Autodesk Inventor part; units mm, degrees
ref_plane "YZ Plane" through (0, 0, 0) normal (1, 0, 0) x (0, 1, 0)
ref_plane "XZ Plane" through (0, 0, 0) normal (0, 1, 0) x (-1, 0, 0)
ref_plane "XY Plane" through (0, 0, 0) normal (0, 0, 1) x (1, 0, 0)
sketch "Sketch1" plane through (0, 0, 0) normal (0, 1, 0) x (-1, 0, 0)
  arc A0 (-85.6318, 54.0093) -> (-85.4518, 52.6798) centre (-90.4518, 52.6798) ccw
  line L0 (-85.6318, 54.0093) -> (-85.6318, 82.6798)
  line L1 (-85.6318, 82.6798) -> (-75.8236, 82.6798)
  line L2 (-75.8236, 82.6798) -> (-75.8236, 52.6798)
  line L3 (-75.8236, 52.6798) -> (-85.4518, 52.6798)
  circle A1 centre (89.5482, 282.6798) radius 5
  circle A2 centre (-90.4518, 282.6798) radius 5
  circle A3 centre (89.5482, 52.6798) radius 5
  circle A4 centre (-15.4518, 247.6798) radius 5
  circle A5 centre (94.5482, 87.6798) radius 5
  circle A6 centre (-15.4518, 87.6798) radius 5
  circle A7 centre (14.5482, 247.6798) radius 5
  circle A8 centre (-95.4518, 247.6798) radius 5
  circle A9 centre (14.5482, 87.6798) radius 5
  circle A10 centre (-95.4518, 87.6798) radius 5
  circle A11 centre (94.5482, 247.6798) radius 5
  line L4 (-25.6318, 52.6798) -> (-35.3318, 52.6798)
  line L5 (-35.3318, 52.6798) -> (-35.3318, 82.6798)
  line L6 (-35.3318, 82.6798) -> (-25.6318, 82.6798)
  line L7 (-25.6318, 82.6798) -> (-25.6318, 52.6798)
  line L8 (24.3682, 82.6798) -> (34.1764, 82.6798)
  line L9 (34.1764, 82.6798) -> (34.1764, 52.6798)
  line L10 (34.1764, 52.6798) -> (24.3682, 52.6798)
  line L11 (24.3682, 52.6798) -> (24.3682, 82.6798)
  line L12 (84.3682, 52.6798) -> (74.6682, 52.6798)
  line L13 (74.6682, 52.6798) -> (74.6682, 82.6798)
  line L14 (74.6682, 82.6798) -> (84.3682, 82.6798)
  line L15 (84.3682, 82.6798) -> (84.3682, 52.6798)
  arc A12 (86.1572, 45.1798) -> (96.0053, 53.4434) centre (86.1572, 55.1798) ccw
  line L16 (96.0053, 53.4434) -> (115.8421, 165.9434)
  arc A13 (115.8421, 165.9434) -> (115.8421, 169.4163) centre (105.994, 167.6798) ccw
  line L17 (115.8421, 169.4163) -> (96.0053, 281.9163)
  arc A14 (96.0053, 281.9163) -> (86.1572, 290.1798) centre (86.1572, 280.1798) ccw
  line L18 (86.1572, 290.1798) -> (-87.0608, 290.1798)
  arc A15 (-87.0608, 290.1798) -> (-96.9089, 281.9163) centre (-87.0608, 280.1798) ccw
  line L19 (-96.9089, 281.9163) -> (-116.7457, 169.4163)
  arc A16 (-116.7457, 169.4163) -> (-116.7457, 165.9434) centre (-106.8976, 167.6798) ccw
  line L20 (-116.7457, 165.9434) -> (-96.9089, 53.4434)
  arc A17 (-96.9089, 53.4434) -> (-87.0608, 45.1798) centre (-87.0608, 55.1798) ccw
  line L21 (-87.0608, 45.1798) -> (86.1572, 45.1798)
  line L22 (12.0482, 180.1798) -> (12.0482, 155.1798)
  line L23 (12.0482, 155.1798) -> (-12.9518, 155.1798)
  line L24 (-12.9518, 155.1798) -> (-12.9518, 180.1798)
  line L25 (-12.9518, 180.1798) -> (12.0482, 180.1798)
  circle A18 centre (25.0482, 100.1798) radius 1.5
  circle A19 centre (25.0482, 230.1798) radius 1.5
  circle A20 centre (-86.9518, 230.1798) radius 1.5
  circle A21 centre (-25.9518, 149.1798) radius 1.5
  circle A22 centre (-25.9518, 100.1798) radius 1.5
  line L26 (-22.4518, 167.6798) -> (-22.4518, 162.6798)
  line L27 (-22.4518, 162.6798) -> (-90.4518, 162.6798)
  line L28 (-90.4518, 162.6798) -> (-90.4518, 167.6798)
  line L29 (-90.4518, 167.6798) -> (-22.4518, 167.6798)
  circle A23 centre (-25.9518, 230.1798) radius 1.5
  circle A24 centre (25.0482, 181.1798) radius 1.5
  circle A25 centre (25.0482, 149.1798) radius 1.5
  circle A26 centre (86.0482, 100.1798) radius 1.5
  circle A27 centre (86.0482, 230.1798) radius 1.5
  circle A28 centre (-86.9518, 181.1798) radius 1.5
  circle A29 centre (-86.9518, 149.1798) radius 1.5
  circle A30 centre (-86.9518, 100.1798) radius 1.5
  circle A31 centre (-25.9518, 181.1798) radius 1.5
  line L30 (89.5482, 167.6798) -> (89.5482, 162.6798)
  line L31 (89.5482, 162.6798) -> (21.5482, 162.6798)
  line L32 (21.5482, 162.6798) -> (21.5482, 167.6798)
  line L33 (21.5482, 167.6798) -> (89.5482, 167.6798)
  circle A32 centre (86.0482, 181.1798) radius 1.5
  circle A33 centre (86.0482, 149.1798) radius 1.5
  circle A34 centre (-65.4518, 267.6798) radius 4
  circle A35 centre (-65.4518, 67.6798) radius 4
  circle A36 centre (64.5482, 267.6798) radius 4
  circle A37 centre (64.5482, 67.6798) radius 4
  point P0 (0, 0)
extrude "Extrusion1" add sketch "Sketch1" along normal blind 5 contours L0 L1 L2 L3 A0 | A1 | A2 | A3 | A4 | A5 | A6 | A7 | A8 | A9 | A10 | A11 | L4 L5 L6 L7 | L8 L9 L10 L11 | L12 L13 L14 L15 | L21 A17 L20 A16 L19 A15 L18 A14 L17 A13 L16 A12 | L22 L23 L24 L25 | A18 | A19 | A20 | A21 | A22 | L26 L27 L28 L29 | A23 | A24 | A25 | A26 | A27 | A28 | A29 | A30 | A31 | L30 L31 L32 L33 | A32 | A33 | A34 | A35 | A36 | A37
sketch "Sketch2" plane through (0, 5, 0) normal (0, 1, 0) x (1, 0, 0)
  arc A0 (85.6318, -54.0093) -> (85.4518, -52.6798) centre (90.4518, -52.6798) ccw
  circle A1 centre (90.4518, -282.6798) radius 5
  circle A2 centre (-89.5482, -52.6798) radius 5
  circle A3 centre (-89.5482, -282.6798) radius 5
  circle A4 centre (90.4518, -52.6798) radius 5
  point P0 (0, 0)
extrude "Extrusion2" cut sketch "Sketch2" against normal through all
sketch "Sketch3" plane through (0, 5, 0) normal (0, 1, 0) x (1, 0, 0)
  line L0 (12.9518, -180.1798) -> (12.9518, -155.1798)
  line L1 (12.9518, -155.1798) -> (-12.0482, -155.1798)
  line L2 (-12.0482, -155.1798) -> (-12.0482, -180.1798)
  line L3 (-12.0482, -180.1798) -> (12.9518, -180.1798)
  point P0 (0, 0)
extrude "Extrusion3" cut sketch "Sketch3" against normal mid plane 50
sketch "Sketch4" plane through (0, 5, 0) normal (0, 1, 0) x (1, 0, 0)
  line L0 (-12.0482, -155.1798) -> (-12.0482, -180.1798)
  line L1 (-12.0482, -180.1798) -> (82.9518, -180.1798)
  line L2 (82.9518, -180.1798) -> (82.9518, -60.1798)
  line L3 (82.9518, -60.1798) -> (-12.0482, -60.1798)
  line L4 (-12.0482, -60.1798) -> (-12.0482, -180.1798)
  line L5 (12.9518, -180.1798) -> (12.9518, -155.1798)
  line L6 (12.9518, -180.1798) -> (-82.0482, -180.1798)
  line L7 (-82.0482, -180.1798) -> (-82.0482, -60.1798)
  line L8 (-82.0482, -60.1798) -> (12.9518, -60.1798)
  line L9 (12.9518, -60.1798) -> (12.9518, -180.1798)
  line L10 (82.9518, -60.1798) -> (-82.0482, -60.1798)
  line L11 (-82.0482, -60.1798) -> (-82.0482, -57.6798)
  line L12 (-82.0482, -57.6798) -> (82.9518, -57.6798)
  line L13 (82.9518, -57.6798) -> (82.9518, -60.1798)
  line L14 (-82.0482, -57.6798) -> (-79.5482, -57.6798)
  line L15 (-79.5482, -57.6798) -> (-79.5482, -180.1798)
  line L16 (-79.5482, -180.1798) -> (-82.0482, -180.1798)
  line L17 (-82.0482, -180.1798) -> (-82.0482, -57.6798)
  line L18 (82.9518, -180.1798) -> (80.4518, -180.1798)
  line L19 (80.4518, -180.1798) -> (80.4518, -57.6798)
  line L20 (80.4518, -57.6798) -> (82.9518, -57.6798)
  line L21 (82.9518, -57.6798) -> (82.9518, -180.1798)
  line L22 (82.9518, -180.1798) -> (-82.0482, -180.1798)
  line L23 (-82.0482, -180.1798) -> (-82.0482, -182.6798)
  line L24 (-82.0482, -182.6798) -> (82.9518, -182.6798)
  line L25 (82.9518, -182.6798) -> (82.9518, -180.1798)
  point P0 (0, 0)
  point P1 (-79.5482, -60.1798)
  point P2 (-12.0482, -60.1798)
  point P3 (80.4518, -60.1798)
  dimension "d6" = 95
  dimension "d7" = 120
  dimension "d8" = 95
  dimension "d9" = 120
  dimension "d10" = 2.5
  dimension "d11" = 2.5
  dimension "d12" = 2.5
  dimension "d13" = 2.5
extrude "Extrusion4" add sketch "Sketch4" along normal blind 50 contours L1 L25 L24 L23 L6 | L8 L15 L12 L19 L3 | L6 L7 L8 L15 | L8 L11 L12 L15 | L19 L3 L2 L1 | L19 L12 L13 L3
sketch "Sketch6" plane through (80.4518, 5, 60.1798) normal (-1, 0, 0) x (0, 0, 1)
  line L0 (122.5, 0) -> (0, 0)
  line L1 (122.5, 0) -> (122.5, 50)
  line L2 (0, 50) -> (122.5, 50)
  line L3 (0, 0) -> (0, 50)
  line L4 (120, 0) -> (120, 50)
  line L5 (0, 0) -> (0, 50)
  line L6 (0, 0) -> (120, 0)
  line L7 (120, 0) -> (120, 5)
  line L8 (120, 5) -> (0, 5)
  line L9 (0, 5) -> (0, 0)
  line L10 (0, 5) -> (120, 0)
  point P0 (-60.1798, -5)
  dimension "d26" = 5
extrude "Extrusion6" add sketch "Sketch6" along normal up to surface (160 mm away) contours L0 L3 L10
sketch "Sketch7" plane through (-79.5482, 10, 60.1798) normal (0, 0.9991, 0.0416) x (1, 0, 0)
  line L0 (67.5, -120.1041) -> (67.5, -95.1258)
  line L1 (67.5, -95.1258) -> (92.5, -95.1258)
  line L2 (92.5, -95.1258) -> (92.5, -120.1041)
  line L3 (160, -118.0226) -> (0, -118.0226)
  point P0 (79.5482, 59.7114)
  point P1 (67.5, -118.0226)
  point P2 (92.5, -118.0226)
extrude "Extrusion7" cut sketch "Sketch7" against normal blind 10
sketch "Sketch8" plane through (-86.1572, 0, 290.1798) normal (0, 0, 1) x (1, 0, 0)
  line L0 (0, 0) -> (173.218, 0)
  line L1 (173.218, 0) -> (173.218, 5)
  line L2 (0, 5) -> (173.218, 5)
  line L3 (0, 0) -> (0, 5)
  line L4 (173.218, 0) -> (173.218, 5)
  line L5 (173.218, 0) -> (115.5513, 0)
  line L6 (115.5513, 0) -> (57.8843, 0)
  line L7 (0, 0) -> (173.218, 0)
  line L8 (0, 0) -> (-9.8481, 0)
  line L9 (0, 0) -> (57.667, 0)
  line L10 (57.667, 0) -> (57.667, 5)
  line L11 (0, 5) -> (173.218, 5)
  line L12 (115.5513, 0) -> (115.5513, 5)
  line L13 (99.109, 5) -> (166.609, 5)
  line L14 (55.167, 7.5) -> (60.167, 7.5)
  line L15 (60.167, 7.5) -> (60.167, 2.5)
  line L16 (60.167, 2.5) -> (55.167, 2.5)
  line L17 (55.167, 2.5) -> (55.167, 7.5)
  line L18 (55.167, 7.5) -> (60.167, 2.5) construction
  line L19 (60.167, 7.5) -> (55.167, 2.5) construction
  line L20 (113.0513, 7.5) -> (118.0513, 7.5)
  line L21 (118.0513, 7.5) -> (118.0513, 2.5)
  line L22 (118.0513, 2.5) -> (113.0513, 2.5)
  line L23 (113.0513, 2.5) -> (113.0513, 7.5)
  line L24 (113.0513, 7.5) -> (118.0513, 2.5) construction
  line L25 (118.0513, 7.5) -> (113.0513, 2.5) construction
  line L26 (60.167, 2.5) -> (62.667, 2.5)
  line L27 (62.667, 2.5) -> (60.167, 5)
  line L28 (55.167, 2.5) -> (52.667, 2.5)
  line L29 (52.667, 2.5) -> (55.167, 5)
  line L30 (118.0513, 2.5) -> (120.5513, 2.5)
  line L31 (120.5513, 2.5) -> (118.0513, 5)
  line L32 (113.0513, 2.5) -> (110.5513, 2.5)
  line L33 (110.5513, 2.5) -> (113.0513, 5)
  point P0 (86.1572, 0)
  dimension "d31" = 57.6667
  dimension "d33" = 57.667
  dimension "d34" = 5
  dimension "d35" = 5
  dimension "d36" = 5
  dimension "d37" = 5
  dimension "d38" = 2.5
  dimension "d39" = 2.5
  dimension "d40" = 2.5
  dimension "d41" = 2.5
extrude "Extrusion8" cut sketch "Sketch8" against normal up to surface (107.5 mm away) contours L16 L17 L2 L10 | L10 L2 L15 L16 | L17 L28 L29 | L15 L27 L26 | L22 L23 L2 L12 | L12 L2 L21 L22 | L21 L31 L30 | L32 L33 L23
properties part number "upper base"
Part model, mm, in its own coordinate system. A direction names the side the tool comes from. Coordinates: 2 decimals unless noted, no trailing zeros. Loops run counter-clockwise (first coordinate to the right, second up) from the corner with the lowest first, then second, coordinate; pieces in that order, holes last. Notation, with made-up numbers: M 54,5 L 94,5 A23 ccw 94,22 Z; hole C 29.5,-20.75 d11. An arc over 180 degrees is marked long. Use a Markdown table: item, result. Add a question column.
Q1. Cut at A-A (y = 33). Write the cut outline in (x, z), and give its area (4 significant figures).
Q2. Which spindle directions (+Z, -Z, +X, -X, +Y, -Y) get a long thin tool onto all of the face, cutting with end or side? Do faces 4 (the flat face through (82.952, 30, 121)), 5 (the flat face through (-82.048, 30, 119)), 6 (the flat face through (-1, 30, 57.68)), 7 (the flat face through (1, 5, 237)). Say none if no direction does.
Q3. Probe L1, parallel to Z at x = 41, y = 29.5; L2, parallel to X at y = 45.5, z = 85; L3, parallel to Y at x = 45, z = 185. List the from-to ranges inside material, lowest first.
Q4. Mould opens along Z. For faces 1 (the cylindrical face through (89.37, 2.54, 287.56)), 2 (the flat face through (106.966, 2.465, 110.481)), 3 (the flat face through (-106.063, 2.465, 224.879)) say: +Z half, -Z half, draft (parallel to the pull), parting line (faces both ways), or undercut.
Q5. Cut at B-B (x = -39). Write the cut outline in (y, z).
Q6. Pin check, flat tips, straight feed: P1, Ø2, axis at x = -59.5, y = 48, coming from the -Z side; P2, Ø5, axis at x = 29, z = 263, coming from the +Y side; P3, Ø3, axis at x = 64, y = 15, coming from the +Z side. Stop position of each tip, or through.
Q7. Cut at C-C (z = 186). Write the cut outline in (x, y), and give its area (3 significant figures).
Worked out:
| question | item | result |
|---|---|---|
| 1 | outline | M -82.05,57.68 L 82.95,57.68 L 82.95,182.68 L -82.05,182.68 Z; hole M -79.55,60.18 L 80.45,60.18 L 80.45,180.18 L -79.55,180.18 Z |
| 1 | area | 1,425 mm2 |
| 2 | face 4 | +Z, -Z, +X, +Y |
| 2 | face 5 | +Z, -Z, -X, +Y |
| 2 | face 6 | -Z, +X, -X, +Y |
| 2 | face 7 | +Z, +X, -X, +Y |
| 3 | L1 | z = 57.68 to 60.18, 180.18 to 182.68 |
| 3 | L2 | x = -82.05 to -79.55, 80.45 to 82.95 |
| 3 | L3 | y = 0 to 5 |
| 4 | face 1 | undercut |
| 4 | face 2 | -Z half |
| 4 | face 3 | +Z half |
| 5 | outline | M 0,45.18 L 5,45.18 L 5,57.68 L 55,57.68 L 55,60.18 L 10,60.18 L 5,180.18 L 55,180.18 L 55,182.68 L 5,182.68 L 5,290.18 L 0,290.18 Z |
| 6 | P1 | stops at z = 57.68 |
| 6 | P2 | stops at y = 5 |
| 6 | P3 | stops at z = 182.68 |
| 7 | outline | M -112.92,0 L 113.82,0 L 113.82,5 L 31.89,5 L 34.39,2.5 L 24.39,2.5 L 26.89,5 L -25.99,5 L -23.49,2.5 L -33.49,2.5 L -30.99,5 L -112.92,5 Z |
| 7 | area | 1,100 mm2 |
